Design review of the part built by this model. Coordinates are the model's own, in mm. A direction names the side the tool comes from. Coordinates: 2 decimals unless noted, no trailing zeros. Loops run counter-clockwise (first coordinate to the right, second up) from the corner with the lowest first, then second, coordinate; pieces in that order, holes last. Notation, with made-up numbers: M -14.5,67.25 L 11.5,67.25 A26 ccw 11.5,81.25 Z; hole C 75,22 d1. An arc over 180 degrees is marked long. One line per item, written item: value.
```python
from build123d import *

# Parameters (mm, degrees)
ESQUISSE1_W             = 4.45
ESQUISSE1_H             = 8
BOSS_EXTRU_1_DEPTH      = 8
ESQUISSE2_R             = 4.597869413
BOSS_EXTRU_2_DEPTH      = 58
ESQUISSE4_R             = 2
ENL_V_MAT_EXTRU_1_DEPTH = 18
ESQUISSE5_R             = 4.597869413
BOSS_EXTRU_3_DEPTH      = 18
BOSS_EXTRU_3_TAPER      = 13


with BuildPart() as part:
    # Esquisse1 → Boss.-Extru.1 (new body)
    with BuildSketch(Plane.XY):
        with Locations((0.087605016, -1.300333333)):
            Rectangle(ESQUISSE1_W, ESQUISSE1_H)
    extrude(amount=BOSS_EXTRU_1_DEPTH)

    # Esquisse2 → Boss.-Extru.2 (add)
    with BuildSketch(Plane.XZ.offset(5.300333333)):
        with Locations(Location((0, 3.983435039, 0), (0, 0, 60.876291729))):
            Circle(ESQUISSE2_R)
    extrude(amount=BOSS_EXTRU_2_DEPTH)

    # Esquisse4 → Enlèv. mat.-Extru.1 (cut)
    with BuildSketch(Plane(origin=(2.312605016, 0, 0), x_dir=(0, 0, -1), z_dir=(1, 0, 0))):
        with Locations(Location((-3.87570667, -0.589342017, 0), (0, 0, 90))):
            Circle(ESQUISSE4_R)
    extrude(amount=-ENL_V_MAT_EXTRU_1_DEPTH, mode=Mode.SUBTRACT)

    # Esquisse5 → Boss.-Extru.3 (add)
    with BuildSketch(Plane.XZ.offset(63.300333333)):
        with Locations(Location((0, 3.983435039, 0), (0, 0, 60.876291729))):
            Circle(ESQUISSE5_R)
    extrude(amount=BOSS_EXTRU_3_DEPTH, taper=BOSS_EXTRU_3_TAPER)


solid = part.part
```
(1) Insertion check: pin 1 (2 mm diameter, centred on x = 0, y = -0.5, fed in from +Z); pin 2 (2 mm diameter, centred on x = -3, y = -34.5, fed in from +Z); pin 3 (0.7 mm diameter, centred on x = 4, z = 5.5, fed in from +Y). Each pin has a flat end and moves straight along its axis. Give the tip position at first contact, or say it passes through.
Reply:
pin 1: stops at z = 8
pin 2: stops at z = 8.12
pin 3: stops at y = -5.3
(2) Tool access review of faces 4 (the flat face through (0, 2.7, 4)), 5 (the flat face through (-2.137, -3, 4)), 6 (the flat face through (0, -1, 0)), 7 (the flat face through (2.313, -3, 4)): name each direction out of +Z, -Z, +X, -X, +Y, -Y from which nothing blocks a thin tool from reaching the whole face with its end or side.
Reply:
face 4: +Z, -Z, +X, -X, +Y
face 5: +Z, -Z, -X, +Y
face 6: -Z, +X, -X, +Y
face 7: +Z, -Z, +X, +Y
(3) Mouldability with a two-part tool opening along Y and no side actions: class faces 1 (the flat face through (3, -5.3, 4)), 2 (the flat face through (0, -1, 8)), 3 (the cylindrical face through (0.119, -1.023, 1.923)) as released by +Y, released by -Y, zero draft, split by the parting line, or undercut.
Reply:
face 1: released by +Y
face 2: zero draft
face 3: undercut
(4) To check wall thickness, follow line 1 along Z through (x, y) = (-1.5, -4); line 2 along X through (y, z) = (-5, 2.5); line 3 along X through (y, z) = (-60, 5). State the ranges of each line that lie inside material, in increasing order. Write a range as [from, to].
Reply:
line 1: z = [0, 8]
line 2: x = [-2.14, 2.31]
line 3: x = [-4.48, 4.48]
(5) We need section A-A on y = -26.5. State the section outline as (x, z) points, then the cut area to 3 significant figures.
Reply:
outline: C 0,3.98 d9.2
area: 66.4 mm2
